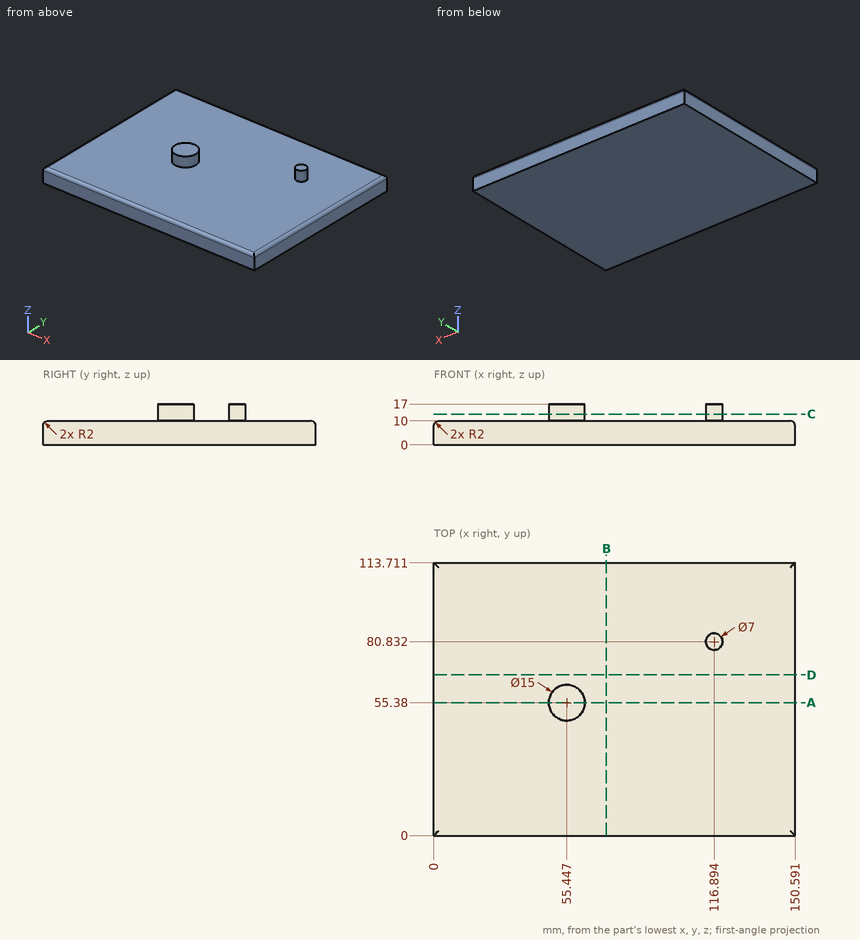
Could you check a few things on this drawing? It's one solid part, dimensions in mm from its lowest x, y, z. Coordinates: 2 decimals unless noted, no trailing zeros. Write each loop counter-clockwise with the first axis right and the second up, starting at its lowest first coordinate (ties: lowest second). Pieces come first, ordered by that corner, then holes. Notation, with made-up numbers: (74, 87) - (97, 87) arc R11 cw to (97, 91) - close; hole circle Ø6 at (10, 85.25). An arc over 180 degrees is marked (long way). Return JSON: item names as keys, results as strings. Group by question number.
Item 1: Please list where these lines run through material, in increasing order: probe 1 along Z at (x, y) = (20, 46.5); probe 2 along X at (y, z) = (86, 8.75).
Item 2: If we section it at B-B (x = 72): Write out the boundary of the cut face in (y, z).
Item 3: If we section it at D-D (y = 67): Write out the boundary of the cut face in (x, z), then the cut area to 3 significant figures.
Item 4: I'm going to push flat-ended pins straight in: pin 1 Ø1.5 at (x, y) = (22, 60) entering from +Z; pin 2 Ø1.5 at (x, z) = (124.5, 10.5) entering from +Y. Where does each tip first touch, or does it pass through?
Item 5: If we section it at C-C (z = 12.75): Write out the boundary of the cut face in (x, y).
Item 6: If we section it at A-A (y = 55.38): Write out the boundary of the cut face in (x, z), then the cut area to 3 significant figures.
Return value:
{
 "1": {"probe 1": "z = 0 to 10", "probe 2": "x = 0.15 to 150.45"},
 "2": {"outline": "(0, 0) - (113.71, 0) - (113.71, 8) arc R2 ccw to (111.71, 10) - (2, 10) arc R2 ccw to (0, 8) - close"},
 "3": {"outline": "(0, 0) - (150.59, 0) - (150.59, 8) arc R2 ccw to (148.59, 10) - (2, 10) arc R2 ccw to (0, 8) - close", "area": "1,500 mm^2"},
 "4": {"pin 1": "stops at z = 10", "pin 2": "stops at y = 112.68"},
 "5": {"outline": "circle Ø15 at (55.45, 55.38); circle Ø7 at (116.89, 80.83)"},
 "6": {"outline": "(0, 0) - (150.59, 0) - (150.59, 8) arc R2 ccw to (148.59, 10) - (62.95, 10) - (62.95, 17) - (47.95, 17) - (47.95, 10) - (2, 10) arc R2 ccw to (0, 8) - close", "area": "1,610 mm^2"}
}
